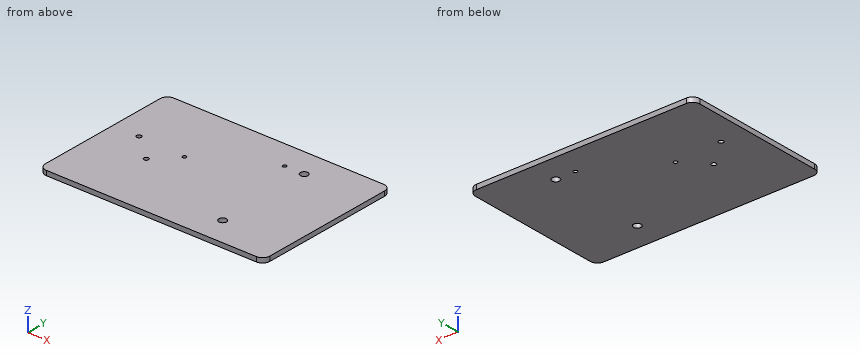
from build123d import *

# Parameters (mm, degrees)
SKETCH1_W           = 152.4
SKETCH1_H           = 101.6
BOSS_EXTRUDE1_DEPTH = 3.175
CUT_EXTRUDE1_REACH  = 5.175
SKETCH2_R           = 2.6
SKETCH2_R_2         = 1.25
SKETCH2_R_3         = 1.5875
FILLET1_R           = 5


with BuildPart() as part:
    # Sketch1 → Boss-Extrude1 (new body)
    with BuildSketch(Plane.XY):
        with Locations((76.2, 50.8)):
            Rectangle(SKETCH1_W, SKETCH1_H)
    extrude(amount=BOSS_EXTRUDE1_DEPTH)

    # Sketch2 → Cut-Extrude1 (cut, up to next)
    with BuildSketch(Plane.XY.offset(3.175), mode=Mode.PRIVATE) as cut_extrude1_sk1:
        with Locations((109.06828742, 18.3)):
            Circle(SKETCH2_R)
    cut_extrude1_tool1 = extrude(cut_extrude1_sk1.sketch, amount=-CUT_EXTRUDE1_REACH, mode=Mode.PRIVATE) & part.part
    add(cut_extrude1_tool1.solids().sort_by_distance((109.068287, 18.3, 3.175))[0], mode=Mode.SUBTRACT)
    # Sketch2 → Cut-Extrude1 (cut, up to next)
    with BuildSketch(Plane.XY.offset(3.175), mode=Mode.PRIVATE) as cut_extrude1_sk2:
        with Locations((109.06828742, 83.3)):
            Circle(SKETCH2_R)
    cut_extrude1_tool2 = extrude(cut_extrude1_sk2.sketch, amount=-CUT_EXTRUDE1_REACH, mode=Mode.PRIVATE) & part.part
    add(cut_extrude1_tool2.solids().sort_by_distance((109.068287, 83.3, 3.175))[0], mode=Mode.SUBTRACT)
    # Sketch2 → Cut-Extrude1 (cut, up to next)
    with BuildSketch(Plane.XY.offset(3.175), mode=Mode.PRIVATE) as cut_extrude1_sk3:
        with Locations((95.79724118, 83.3)):
            Circle(SKETCH2_R_2)
    cut_extrude1_tool3 = extrude(cut_extrude1_sk3.sketch, amount=-CUT_EXTRUDE1_REACH, mode=Mode.PRIVATE) & part.part
    add(cut_extrude1_tool3.solids().sort_by_distance((95.797241, 83.3, 3.175))[0], mode=Mode.SUBTRACT)
    # Sketch2 → Cut-Extrude1 (cut, up to next)
    with BuildSketch(Plane.XY.offset(3.175), mode=Mode.PRIVATE) as cut_extrude1_sk4:
        with Locations((49.94724118, 57.26)):
            Circle(SKETCH2_R_2)
    cut_extrude1_tool4 = extrude(cut_extrude1_sk4.sketch, amount=-CUT_EXTRUDE1_REACH, mode=Mode.PRIVATE) & part.part
    add(cut_extrude1_tool4.solids().sort_by_distance((49.947241, 57.26, 3.175))[0], mode=Mode.SUBTRACT)
    # Sketch2 → Cut-Extrude1 (cut, up to next)
    with BuildSketch(Plane.XY.offset(3.175), mode=Mode.PRIVATE) as cut_extrude1_sk5:
        with Locations((17.879257387, 58.74)):
            Circle(SKETCH2_R_3)
    cut_extrude1_tool5 = extrude(cut_extrude1_sk5.sketch, amount=-CUT_EXTRUDE1_REACH, mode=Mode.PRIVATE) & part.part
    add(cut_extrude1_tool5.solids().sort_by_distance((17.879257, 58.74, 3.175))[0], mode=Mode.SUBTRACT)
    # Sketch2 → Cut-Extrude1 (cut, up to next)
    with BuildSketch(Plane.XY.offset(3.175), mode=Mode.PRIVATE) as cut_extrude1_sk6:
        with Locations((36.299257387, 42.86)):
            Circle(SKETCH2_R_3)
    cut_extrude1_tool6 = extrude(cut_extrude1_sk6.sketch, amount=-CUT_EXTRUDE1_REACH, mode=Mode.PRIVATE) & part.part
    add(cut_extrude1_tool6.solids().sort_by_distance((36.299257, 42.86, 3.175))[0], mode=Mode.SUBTRACT)

    # Fillet1
    fillet1_edges = [part.edges().sort_by_distance(p)[0] for p in [
        (0, 101.6, 1.5875),
        (152.4, 101.6, 1.5875),
        (152.4, 0, 1.5875),
        (0, 0, 1.5875),
    ]]
    fillet(fillet1_edges, radius=FILLET1_R)


solid = part.part
The listing builds one solid part. Answer for the finished solid, in the listing's coordinates (mm). Give positions to 0.01 mm unless a question says otherwise; leave off trailing zeros. Write each loop counter-clockwise with the first axis right and the second up, starting at its lowest first coordinate (ties: lowest second). Pieces come first, ordered by that corner, then holes.
Item 1: Section A-A, the plane y = 18.3 is taken. Write down the section's boundary in (x, z) (3 decimals).
Item 2: Section B-B, the plane y = 42.86 is taken. Write down the section's boundary in (x, z) (3 decimals).
Item 3: Find the intervals of material crossed by line 1 along X through (y, z) = (18, 0.85); line 2 along X through (y, z) = (16.5, 0.6); line 3 along Y through (x, z) = (17, 1.6), in increasing order.
Completed:
1. outline: (0, 0) - (106.468, 0) - (106.468, 3.175) - (0, 3.175) - close; (111.668, 0) - (152.4, 0) - (152.4, 3.175) - (111.668, 3.175) - close
2. outline: (0, 0) - (34.712, 0) - (34.712, 3.175) - (0, 3.175) - close; (37.887, 0) - (152.4, 0) - (152.4, 3.175) - (37.887, 3.175) - close
3. line 1: x = 0 to 106.49, 111.65 to 152.4
3. line 2: x = 0 to 107.19, 110.94 to 152.4
3. line 3: y = 0 to 57.42, 60.06 to 101.6
